Verification items for the finished model (mm, model axes). A direction names the side the tool comes from. Give positions to 0.01 mm unless a question says otherwise; leave off trailing zeros. Write each loop counter-clockwise with the first axis right and the second up, starting at its lowest first coordinate (ties: lowest second). Pieces come first, ordered by that corner, then holes. Notation, with made-up numbers: (-31.5, 48) - (-14.5, 48) arc R19 cw to (-14.5, 82) - close; hole circle Ø9 at (49.25, 55). An arc over 180 degrees is marked (long way). Answer as a JSON object with one key per item and string values. Group by question number.
Item 1: Draft check along Z on faces 1 (the face through (3.3, -17, -2.4)), 2 (the face through (0, -16, -6)), 3 (the face through (0, 16, 2)). Enter one of: +Z half, -Z half, draft (parallel to the pull), parting line (faces both ways), or undercut.
Item 2: Tool access check on faces 4 (the face through (0, 1, 0)), 5 (the face through (-5.75, -0.3, 2.5)), 6 (the face through (-7.25, -4, 1)), 7 (the face through (0, 12, 1)), 8 (the face through (0, -7, 2)). Record the directions out of +Z, -Z, +X, -X, +Y, -Y that give a thin tool (end or side, any length) a straight path to the whole face; none if there is none.
Item 3: Scan lines: line 1 along Y through (x, z) = (0, 1.55); line 2 along Z through (x, y) = (4.25, -16.85); line 3 along Y through (x, z) = (3, 1.25). Record each from-to range of solid material in increasing order. Write a range as [from, to].
Item 4: Go/stop test with flat-tipped pins: pin 1 (3 mm diameter, centred on x = 0, y = 14, fed in from +Z); pin 2 (1 mm diameter, centred on x = -2.5, y = -3, fed in from -Z); pin 3 (3 mm diameter, centred on x = -4.25, z = -2.4, fed in from -Y); pin 4 (2.5 mm diameter, centred on x = 0, z = -10, fed in from +Y). Record where each tip stops, or that it passes through.
Item 5: Sectioned sample at D-D, the plane z = -10. Record the boundary of the cut face in (x, y).
Item 6: Sectioned sample at B-B, the plane x = -4.25. Record the boundary of the cut face in (y, z).
Item 7: Sectioned sample at C-C, the plane x = 2.5. Record the boundary of the cut face in (y, z).
Item 8: Sectioned sample at A-A, the plane y = 14. Record the boundary of the cut face in (x, z).
```python
from build123d import *

# Parameters (mm, degrees)
SKETCH1_W           = 14.5
SKETCH1_H           = 36
BOSS_EXTRUDE1_DEPTH = 4
SKETCH3_W           = 14.5
SKETCH3_H           = 16
BOSS_EXTRUDE2_DEPTH = 2
SKETCH2_W           = 11.5
SKETCH2_H           = 36
CUT_EXTRUDE1_DEPTH  = 2
SKETCH4_R           = 0.95
CUT_EXTRUDE2_DEPTH  = 15
SKETCH5_W           = 11.5
SKETCH5_H           = 9
CUT_EXTRUDE3_DEPTH  = 15
SKETCH6_R           = 0.95
CUT_EXTRUDE4_DEPTH  = 3


with BuildPart() as part:
    # Sketch1 → Boss-Extrude1 (new body)
    with BuildSketch(Plane.XY):
        Rectangle(SKETCH1_W, SKETCH1_H)
    extrude(amount=BOSS_EXTRUDE1_DEPTH)

    # Sketch3 → Boss-Extrude2 (add)
    with BuildSketch(Plane.XZ.offset(18)):
        with Locations((0, -4)):
            Rectangle(SKETCH3_W, SKETCH3_H)
    extrude(amount=-BOSS_EXTRUDE2_DEPTH)

    # Sketch2 → Cut-Extrude1 (cut)
    with BuildSketch(Plane.XY.offset(4)):
        Rectangle(SKETCH2_W, SKETCH2_H)
    extrude(amount=-CUT_EXTRUDE1_DEPTH, mode=Mode.SUBTRACT)

    # Sketch4 → Cut-Extrude2 (cut, through all)
    with BuildSketch(Plane.XY.offset(2)):
        with Locations((0, -14)):
            Circle(SKETCH4_R)
        with Locations((0, 14)):
            Circle(SKETCH4_R)
    extrude(amount=-CUT_EXTRUDE2_DEPTH, mode=Mode.SUBTRACT)

    # Sketch5 → Cut-Extrude3 (cut, through all)
    with BuildSketch(Plane.XY.offset(2)):
        with Locations((0, 7.5)):
            Rectangle(SKETCH5_W, SKETCH5_H)
    extrude(amount=-CUT_EXTRUDE3_DEPTH, mode=Mode.SUBTRACT)

    # Sketch6 → Cut-Extrude4 (cut, through all)
    with BuildSketch(Plane(origin=(0, -16, 0), x_dir=(1, 0, 0), z_dir=(0, 1, 0))):
        with Locations((-4.25, 2.395194775)):
            Circle(SKETCH6_R)
        with Locations((4.25, 2.395194775)):
            Circle(SKETCH6_R)
        with Locations((0, 10)):
            Circle(SKETCH6_R)
    extrude(amount=-CUT_EXTRUDE4_DEPTH, mode=Mode.SUBTRACT)


solid = part.part
```
Geometry check:
{
 "1": {"face 1": "undercut", "face 2": "draft", "face 3": "+Z half"},
 "2": {"face 4": "-Z, +X, -X, +Y", "face 5": "+Z", "face 6": "+Z, -Z, -X, +Y, -Y", "face 7": "+Z, -Z", "face 8": "+Z, +Y, -Y"},
 "3": {"line 1": "[-18, -14.95], [-13.05, 3], [12, 13.05], [14.95, 18]", "line 2": "[-12, -3.35], [-1.45, 2]", "line 3": "[-18, 3], [12, 18]"},
 "4": {"pin 1": "z = 2", "pin 2": "z = 0", "pin 3": "y = -18", "pin 4": "y = -16"},
 "5": {"outline": "(-7.25, -18) - (-0.95, -18) - (-0.95, -16) - (-7.25, -16) - close; (0.95, -18) - (7.25, -18) - (7.25, -16) - (0.95, -16) - close"},
 "6": {"outline": "(-18, -12) - (-16, -12) - (-16, -3.35) - (-18, -3.35) - close; (-18, -1.45) - (-16, -1.45) - (-16, 0) - (3, 0) - (3, 2) - (-18, 2) - close; (12, 0) - (18, 0) - (18, 2) - (12, 2) - close"},
 "7": {"outline": "(-18, -12) - (-16, -12) - (-16, 0) - (3, 0) - (3, 2) - (-18, 2) - close; (12, 0) - (18, 0) - (18, 2) - (12, 2) - close"},
 "8": {"outline": "(-7.25, 0) - (-0.95, 0) - (-0.95, 2) - (-5.75, 2) - (-5.75, 4) - (-7.25, 4) - close; (0.95, 0) - (7.25, 0) - (7.25, 4) - (5.75, 4) - (5.75, 2) - (0.95, 2) - close"}
}
